Can you work these out from the drawing? Everything is in mm from the part's minimum corner. A direction names the side the tool comes from. Coordinates: 2 decimals unless noted, no trailing zeros. Order: outer loops, then holes, each group sorted by start corner. A loop starts at its lowest first (then second) coordinate and runs counter-clockwise, first axis right, second up. Notation, with made-up numbers: (1.25, 27.25) - (51.25, 27.25) arc R13 ccw to (51.25, 44.25) - close; hole circle Ø11 at (-10, 64). An arc over 180 degrees is marked (long way). Answer as CSV lines item,"result". Start each with the question number.
Q1. For pin 1 Ø5.5 at (x, y) = (65, 35) entering from +Z; pin 2 Ø3 at (y, z) = (28, 4) entering from -X, each with a flat end and sliding along its axis, tell me the tip position at first contact or that it passes through.
Q2. For the marked faces 4 and 5, which set-ups out of +Z, -Z, +X, -X, +Y, -Y let a thin tool reach every point of the face, with its end or its side?
Q3. Suppose I cut it at B-B (x = 35). Please give me the cut outline in (y, z).
Q4. Thinking about a two-plate mould opening in Y: for the marked faces 1, 2 and 3, which applies, released by +Y, released by -Y, zero draft, split by the parting line, or undercut?
Q5. Suppose I cut it at C-C (z = 1.75). Please give me the cut outline in (x, y).
Q6. Suppose I cut it at A-A (y = 44). Please give me the cut outline in (x, z), then the cut area to 3 significant figures.
Q7. Suppose I cut it at D-D (x = 5). Please give me the cut outline in (y, z).
Q8. I need wall thicknesses on line 1 (X direction, y = 65, z = 2.25); line 2 (Y direction, x = 5, z = 4.5); line 3 (X direction, y = 45, z = 3). Which ranges of each line are inside material? Lowest first, please.
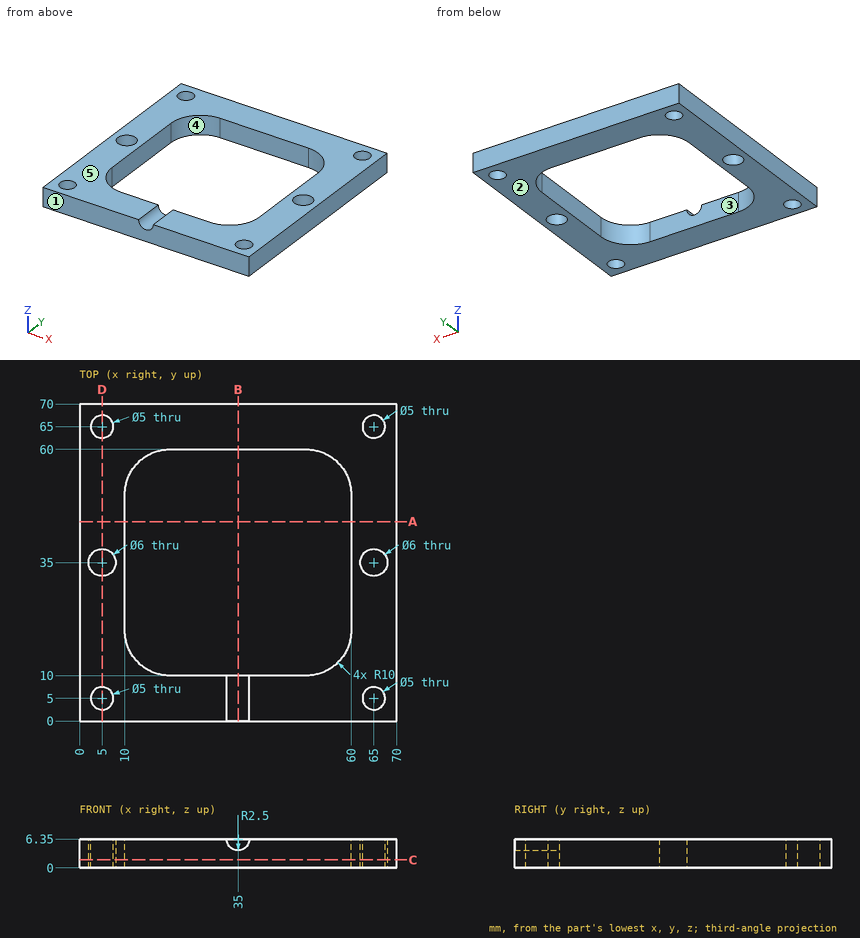
Here are the results:
1,pin 1,"passes through"
1,pin 2,"stops at x = 0"
2,face 4,"+Z, -Z"
2,face 5,"+Z, +X, -X, +Y, -Y"
3,outline,"(0, 0) - (10, 0) - (10, 3.85) - (0, 3.85) - close; (60, 0) - (70, 0) - (70, 6.35) - (60, 6.35) - close"
4,face 1,"released by -Y"
4,face 2,"zero draft"
4,face 3,"undercut"
5,outline,"(0, 0) - (70, 0) - (70, 70) - (0, 70) - close; hole circle Ø6 at (5, 35); hole circle Ø5 at (5, 5); hole circle Ø5 at (5, 65); hole (10, 20) arc R10 ccw to (20, 10) - (50, 10) arc R10 ccw to (60, 20) - (60, 50) arc R10 ccw to (50, 60) - (20, 60) arc R10 ccw to (10, 50) - close; hole circle Ø6 at (65, 35); hole circle Ø5 at (65, 5); hole circle Ø5 at (65, 65)"
6,outline,"(0, 0) - (10, 0) - (10, 6.35) - (0, 6.35) - close; (60, 0) - (70, 0) - (70, 6.35) - (60, 6.35) - close"
6,area,"127 mm²"
7,outline,"(0, 0) - (2.5, 0) - (2.5, 6.35) - (0, 6.35) - close; (7.5, 0) - (32, 0) - (32, 6.35) - (7.5, 6.35) - close; (38, 0) - (62.5, 0) - (62.5, 6.35) - (38, 6.35) - close; (67.5, 0) - (70, 0) - (70, 6.35) - (67.5, 6.35) - close"
8,line 1,"x = 0 to 2.5, 7.5 to 62.5, 67.5 to 70"
8,line 2,"y = 0 to 2.5, 7.5 to 32, 38 to 62.5, 67.5 to 70"
8,line 3,"x = 0 to 10, 60 to 70"
